```python
from build123d import *

# Parameters (mm, degrees)
F1_DEPTH = 25.4


with BuildPart() as f1:
    # F0 (on Right) → F1 (new body)
    with BuildSketch(Plane.YZ):
        Polygon((812.8, 112.629811), (812.8, 163.429811), (-812.8, 163.429811), (-812.8, 112.629811), (-579.4375, 112.629811), (-234.009025, 112.629811), (-118.2624, 112.629811), (118.2624, 112.629811), (234.009025, 112.629811), (579.4375, 112.629811), align=None)
        Polygon((-118.2624, 112.629811), (-234.009025, 112.629811), (-371.145546, 45.64588), (-695.184125, -112.629811), (-579.4375, -112.629811), align=None)
        Polygon((579.4375, -56.093712), (234.009025, 112.629811), (118.2624, 112.629811), (579.4375, -112.629811), (695.184125, -112.629811), align=None)
        Polygon((695.184125, -112.629811), (579.4375, -112.629811), (118.2624, -112.629811), (-118.2624, -112.629811), (-579.4375, -112.629811), (-695.184125, -112.629811), (-812.8, -112.629811), (-812.8, -163.429811), (812.8, -163.429811), (812.8, -112.629811), align=None)
    extrude(amount=F1_DEPTH)


solid = f1.part
```
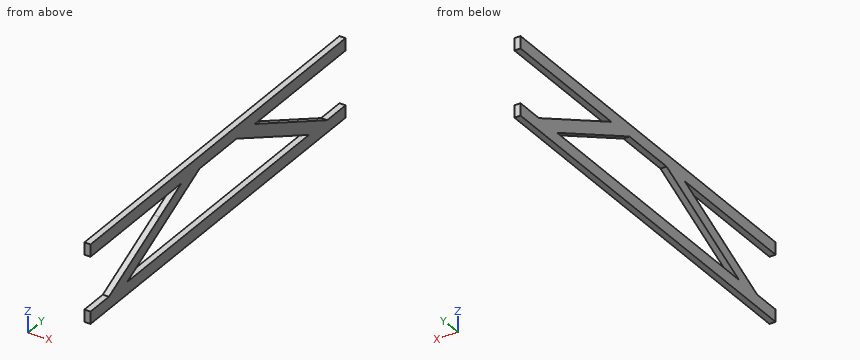
Verification items for the finished model (mm, model axes). Give positions to 0.01 mm unless a question says otherwise; leave off trailing zeros. Order: outer loops, then holes, each group sorted by start corner. A loop starts at its lowest first (then second) coordinate and runs counter-clockwise, first axis right, second up. Notation, with made-up numbers: (50.25, 85) -> (81.25, 85) arc R5 ccw to (81.25, 92) -> close; hole circle Ø8 at (79, 43.5). An arc over 180 degrees is marked (long way). Use a Markdown table: item, result.
1) Material ranges on probe 1 along Z at (x, y) = (4.5, -579); probe 2 along Z at (x, y) = (17, 414.5); probe 3 along Y at (x, z) = (14.5, -92.5), recorded low to high.
Results:
| item | result |
|---|---|
| probe 1 | -163.43 to -112.63, -112.42 to -55.88, 112.63 to 163.43 |
| probe 2 | -163.43 to -112.63, -32.07 to 24.47, 112.63 to 163.43 |
| probe 3 | -653.97 to -538.23, 538.23 to 653.97 |
2) Depth check by flat-ended pin: pin 1 Ø12 at (x, z) = (11, 57.5) entering from -Y; pin 2 Ø2 at (x, z) = (3.5, 14) entering from -Y; pin 3 Ø6 at (y, z) = (-593.5, -94) entering from -X; pin 4 Ø3 at (x, z) = (19.5, 9) entering from -Y. Enter the tip coordinate at first touch or a pass-through.
Results:
| item | result |
|---|---|
| pin 1 | y = -359.16 |
| pin 2 | y = -437.98 |
| pin 3 | x = 0 |
| pin 4 | y = -449.24 |
3) Section check A-A, the plane y = -56. Record the boundary of the cut face in (x, z).
Results:
| item | result |
|---|---|
| outline | (0, -163.43) -> (25.4, -163.43) -> (25.4, -112.63) -> (0, -112.63) -> close; (0, 112.63) -> (25.4, 112.63) -> (25.4, 163.43) -> (0, 163.43) -> close |
4) Section check B-B, the plane x = 4.75. Record the boundary of the cut face in (y, z), then the cut area to 3 significant figures.
Results:
| item | result |
|---|---|
| outline | (-812.8, -163.43) -> (812.8, -163.43) -> (812.8, -112.63) -> (695.18, -112.63) -> (234.01, 112.63) -> (812.8, 112.63) -> (812.8, 163.43) -> (-812.8, 163.43) -> (-812.8, 112.63) -> (-234.01, 112.63) -> (-695.18, -112.63) -> (-812.8, -112.63) -> close; hole (-579.44, -112.63) -> (579.44, -112.63) -> (118.26, 112.63) -> (-118.26, 112.63) -> close |
| area | 217,000 mm² |
5) Section check C-C, the plane z = 27. Record the boundary of the cut face in (x, y), then the cut area to 3 significant figures.
Results:
| item | result |
|---|---|
| outline | (0, -409.32) -> (25.4, -409.32) -> (25.4, -293.57) -> (0, -293.57) -> close; (0, 293.57) -> (25.4, 293.57) -> (25.4, 409.32) -> (0, 409.32) -> close |
| area | 5,880 mm² |
6) Section check D-D, the plane y = 478.5. Record the boundary of the cut face in (x, z), then the cut area to 3 significant figures.
Results:
| item | result |
|---|---|
| outline | (0, -163.43) -> (25.4, -163.43) -> (25.4, -112.63) -> (0, -112.63) -> close; (0, -63.33) -> (25.4, -63.33) -> (25.4, -6.79) -> (0, -6.79) -> close; (0, 112.63) -> (25.4, 112.63) -> (25.4, 163.43) -> (0, 163.43) -> close |
| area | 4,020 mm² |
